from build123d import *

# Parameters (mm, degrees)
BOSS_EXTRUDE1_DEPTH     = 64
CUT_EXTRUDE1_DEPTH      = 61
CUT_EXTRUDE2_DEPTH      = 103.493902258
CUT_EXTRUDE2_DEPTH_BACK = 103.493902258
CUT_EXTRUDE3_DEPTH      = 43
CUT_EXTRUDE4_DEPTH      = 105.961897849
CHAMFER1_SIZE           = 1
SKETCH6_R               = 2.2
CUT_EXTRUDE5_DEPTH      = 94.648278148
BOSS_EXTRUDE2_DEPTH     = 14
CUT_EXTRUDE6_DEPTH      = 106.81625079
SKETCH9_R               = 1.85
CUT_EXTRUDE7_DEPTH      = 93.746967605
FILLET1_R               = 2
FILLET2_R               = 12
SKETCH10_R              = 2.2
CUT_EXTRUDE8_DEPTH      = 108.168092266
FILLET3_R               = 5
FILLET4_START           = 44
FILLET4_DEPTH           = 31
SKETCH11_R              = 2.2
CUT_EXTRUDE9_DEPTH      = 97.098348533
SKETCH12_W              = 18
SKETCH12_H              = 23
CUT_EXTRUDE10_DEPTH     = 22
CUT_EXTRUDE11_REACH     = 95.568
SKETCH13_R              = 1.500000659
SKETCH13_R_2            = 1.499999352


with BuildPart() as part:
    # Sketch1 → Boss-Extrude1 (new body)
    with BuildSketch(Plane.XY):
        with BuildLine():
            Line((-14, 0), (-14, 75))
            Line((-14, 75), (36, 75))
            Line((36, 75), (36, 44))
            Line((36, 44), (14, 44))
            Line((14, 44), (14, 0))
            ThreePointArc((14, 0), (0, -14), (-14, 0))
        make_face()
    extrude(amount=BOSS_EXTRUDE1_DEPTH)

    # Sketch2 → Cut-Extrude1 (cut)
    with BuildSketch(Plane(origin=(0, 75, 0), x_dir=(1, 0, 0), z_dir=(0, 1, 0))):
        Polygon((-11, 0), (-11, -12), (-5, -18), (5, -18), (11, -12), (11, 0), align=None)
    extrude(amount=-CUT_EXTRUDE1_DEPTH, mode=Mode.SUBTRACT)

    # Sketch3 → Cut-Extrude2 (cut, two sides: drawn at the far end of the back side and taken through both)
    with BuildSketch(Plane(origin=(14, 0, 0), x_dir=(0, 0, -1), z_dir=(1, 0, 0)).offset(-CUT_EXTRUDE2_DEPTH_BACK)):
        Polygon((-64, 14), (-41, 34), (-41, 75), (-64, 75), align=None)
    extrude(amount=CUT_EXTRUDE2_DEPTH + CUT_EXTRUDE2_DEPTH_BACK, mode=Mode.SUBTRACT)

    # Sketch4 → Cut-Extrude3 (cut)
    with BuildSketch(Plane.XY.offset(64)):
        Polygon((-10.2, 14), (-10.2, 75), (36, 75), (36, 48), (10.2, 48), (10.2, 14), align=None)
    extrude(amount=-CUT_EXTRUDE3_DEPTH, mode=Mode.SUBTRACT)

    # Sketch5 → Cut-Extrude4 (cut, through all)
    with BuildSketch(Plane.XY.offset(64)):
        with BuildLine():
            Line((-0.5, -10.438031424), (-0.5, -13.99106858))
            ThreePointArc((-0.5, -13.99106858), (0, -14), (0.5, -13.99106858))
            Line((0.5, -13.99106858), (0.5, -10.438031424))
            ThreePointArc((0.5, -10.438031424), (0, 10.45), (-0.5, -10.438031424))
        make_face()
    extrude(amount=-CUT_EXTRUDE4_DEPTH, mode=Mode.SUBTRACT)

    # Chamfer1
    chamfer1_edges = [part.edges().sort_by_distance(p)[0] for p in [
        (0, 10.45, 0),
        (0, 10.45, 64),
    ]]
    chamfer(chamfer1_edges, length=CHAMFER1_SIZE)

    # Sketch6 → Cut-Extrude5 (cut, through all)
    with BuildSketch(Plane.XY.offset(21)):
        with Locations((0, 62)):
            Circle(SKETCH6_R)
        with Locations((0, 27)):
            Circle(SKETCH6_R)
        with Locations((25, 58)):
            Circle(SKETCH6_R)
    extrude(amount=-CUT_EXTRUDE5_DEPTH, mode=Mode.SUBTRACT)

    # Sketch7 → Boss-Extrude2 (add)
    with BuildSketch(Plane(origin=(-14, 0, 0), x_dir=(0, 0, -1), z_dir=(1, 0, 0))):
        Polygon((-41, 62.2), (-21, 62.2), (-21, 60.2), (-39, 60.2), (-39, 44.2), (-21, 44.2), (-21, 42.2), (-41, 42.2), align=None)
    extrude(amount=-BOSS_EXTRUDE2_DEPTH)

    # Sketch8 → Cut-Extrude6 (cut, through all)
    with BuildSketch(Plane(origin=(0, 62.2, 0), x_dir=(1, 0, 0), z_dir=(0, 1, 0))):
        Polygon((-14, -21), (-28, -39), (-28, -21), align=None)
    extrude(amount=-CUT_EXTRUDE6_DEPTH, mode=Mode.SUBTRACT)

    # Sketch9 → Cut-Extrude7 (cut, through all)
    with BuildSketch(Plane.XY.offset(41)):
        with Locations((-22, 52.2)):
            Circle(SKETCH9_R)
    extrude(amount=-CUT_EXTRUDE7_DEPTH, mode=Mode.SUBTRACT)

    # Fillet1
    fillet1_edges = [part.edges().sort_by_distance(p)[0] for p in [
        (-28, 42.2, 40),
        (-28, 62.2, 40),
    ]]
    fillet(fillet1_edges, radius=FILLET1_R)

    # Fillet2
    fillet2_edges = [part.edges().sort_by_distance(p)[0] for p in [
        (-12.5, 75, 0),
        (-12.1, 75, 41),
    ]]
    fillet(fillet2_edges, radius=FILLET2_R)

    # Sketch10 → Cut-Extrude8 (cut, through all)
    with BuildSketch(Plane(origin=(14, 0, 0), x_dir=(0, 0, -1), z_dir=(1, 0, 0))):
        with Locations(Location((-31, 33, 0), (0, 0, 90))):
            Circle(SKETCH10_R)
    extrude(amount=-CUT_EXTRUDE8_DEPTH, mode=Mode.SUBTRACT)

    # Fillet3
    fillet3_edges = [part.edges().sort_by_distance(p)[0] for p in [
        (36, 46, 41),
    ]]
    fillet(fillet3_edges, radius=FILLET3_R)

    # Fillet4: read off the stored shape, not the designer's step
    # Fillet4 outline → Fillet4 (cut)
    with BuildSketch(Plane(origin=(0, 0, 0), x_dir=(1, 0, 0), z_dir=(0, 1, 0)).offset(FILLET4_START)):
        with BuildLine():
            ThreePointArc((18, 0), (30.727922061, -5.272077939), (36, -18))
            Line((36, -18), (36, 0))
            Line((36, 0), (18, 0))
        make_face()
    extrude(amount=FILLET4_DEPTH, mode=Mode.SUBTRACT)

    # Sketch11 → Cut-Extrude9 (cut, through all)
    with BuildSketch(Plane(origin=(0, 48, 0), x_dir=(1, 0, 0), z_dir=(0, 1, 0))):
        with Locations(Location((24, -31, 0), (0, 0, 270))):
            Circle(SKETCH11_R)
    extrude(amount=-CUT_EXTRUDE9_DEPTH, mode=Mode.SUBTRACT)

    # Sketch12 → Cut-Extrude10 (cut)
    with BuildSketch(Plane.ZY.offset(-36)):
        with Locations((9, 59.5)):
            Rectangle(SKETCH12_W, SKETCH12_H)
    extrude(amount=CUT_EXTRUDE10_DEPTH, mode=Mode.SUBTRACT)

    # Sketch13 → Cut-Extrude11 (cut, up to next)
    with BuildSketch(Plane.XZ.offset(-44), mode=Mode.PRIVATE) as cut_extrude11_sk1:
        with Locations((19.000002521, 8.999996593)):
            Circle(SKETCH13_R)
    cut_extrude11_tool1 = extrude(cut_extrude11_sk1.sketch, amount=-CUT_EXTRUDE11_REACH, mode=Mode.PRIVATE) & part.part
    # Sketch13 → Cut-Extrude11 (cut, up to next)
    with BuildSketch(Plane.XZ.offset(-44), mode=Mode.PRIVATE) as cut_extrude11_sk2:
        with Locations((27.000001248, 8.999995496)):
            Circle(SKETCH13_R_2)
    cut_extrude11_tool2 = extrude(cut_extrude11_sk2.sketch, amount=-CUT_EXTRUDE11_REACH, mode=Mode.PRIVATE) & part.part
    add(cut_extrude11_tool1.solids().sort_by_distance((19.000003, 44, 8.999997))[0], mode=Mode.SUBTRACT)
    add(cut_extrude11_tool2.solids().sort_by_distance((27.000001, 44, 8.999995))[0], mode=Mode.SUBTRACT)


solid = part.part
Source: CAD feature listing. Evaluate the final solid. Frame: model axes, mm. A direction names the side the tool comes from. Coordinates: 2 decimals unless noted, no trailing zeros. Loops run counter-clockwise (first coordinate to the right, second up) from the corner with the lowest first, then second, coordinate; pieces in that order, holes last. Notation, with made-up numbers: (-25, 3.5) -> (-16, 3.5) arc R14 cw to (-16, 11.5) -> close; hole circle Ø4 at (28.5, 72.25). An arc over 180 degrees is marked (long way). Answer in a Markdown table with one row per item. Add a question column.
Q1. Pull-direction query (X, two-part tool) for faces 4 (the face through (-8, 45, 15)), 5 (the face through (14, 60, 9)), 6 (the face through (-10.2, 37, 33)), 7 (the face through (23.3, 48, 33.4)); classes: pulls with the +X half, pulls with the -X half, needs draft (parallel to the pull), parting line crosses it, or undercut.
Q2. Contact query for flat-ended pins moving along their axis: pin 1 Ø4 at (y, z) = (52.5, 11.5) entering from -X; pin 2 Ø4 at (x, y) = (-11.5, 36.5) entering from +Z; pin 3 Ø7 at (y, z) = (33, 31) entering from +X; pin 4 Ø4 at (y, z) = (33, 31) entering from +X. Output: stop coordinate, or through.
Q3. Section B-B on z = 31. Give the number of separate pieces and of enclosed holes in the cut face, and give its area (3 significant figures).
Q4. Section C-C on x = -17. Return the cut outline in (y, z), and give its area (3 significant figures).
Q5. Reachability of faces 1 (the face through (-19, 42.2, 33)), 2 (the face through (23, 71, 11)), 3 (the face through (25, 44, 20)) from +Z, -Z, +X, -X, +Y, -Y: full face, straight path, thin tool, end or side. Return the list, or none.
Q6. Section A-A on y = 52.2. Return the cut outline in (x, z), and give its area (3 significant figures).
Q7. Section D-D on z = 5. Return the cut outline in (x, y).
Q8. Ray query, line 1 along Y through (x, z) = (23, 12.5); line 2 along Y through (x, z) = (-22, 39.5); line 3 along X through (y, z) = (21.5, 7). Return the intervals inside material, ascending.
Computed values:
| question | item | result |
|---|---|---|
| 1 | face 4 | undercut |
| 1 | face 5 | pulls with the +X half |
| 1 | face 6 | undercut |
| 1 | face 7 | needs draft |
| 2 | pin 1 | stops at x = -14 |
| 2 | pin 2 | stops at z = 41 |
| 2 | pin 3 | stops at x = 14 |
| 2 | pin 4 | passes through |
| 3 | separate pieces | 4 |
| 3 | enclosed holes | 0 |
| 3 | area | 782 mm^2 |
| 4 | outline | (42.2, 24.86) -> (44.2, 24.86) -> (44.2, 39) -> (60.2, 39) -> (60.2, 24.86) -> (62.2, 24.86) -> (62.2, 41) -> (42.2, 41) -> close |
| 4 | area | 96.6 mm^2 |
| 5 | face 1 | +Z, -Z, -X, -Y |
| 5 | face 2 | -Z, +X |
| 5 | face 3 | +Z, -Z, +X, -Y |
| 6 | outline | (-28, 39) -> (-23.85, 39) -> (-23.85, 41) -> (-28, 41) -> close; (-20.15, 39) -> (-14, 39) -> (-14, 0) -> (-11, 0) -> (-11, 12) -> (-5, 18) -> (5, 18) -> (11, 12) -> (11, 0) -> (14, 0) -> (14, 18) -> (36, 18) -> (36, 21) -> (-10.2, 21) -> (-10.2, 41) -> (-20.15, 41) -> close |
| 6 | area | 391 mm^2 |
| 7 | outline | (-14, 0) arc R14 ccw to (-0.5, -13.99) -> (-0.5, -10.44) arc R10.45 cw (long way) to (0.5, -10.44) -> (0.5, -13.99) arc R14 ccw to (14, 0) -> (14, 44) -> (30.45, 44) -> (30.45, 48) -> (14, 48) -> (14, 71) -> (30.45, 71) -> (30.45, 75) -> (11, 75) -> (11, 14) -> (-11, 14) -> (-11, 72.75) -> (-14, 72.75) -> close |
| 8 | line 1 | y = 44 to 48, 71 to 75 |
| 8 | line 2 | y = 42.2 to 50.35, 54.05 to 62.2 |
| 8 | line 3 | x = -14 to -11, 11 to 14 |
